```python
from build123d import *

# Parameters (mm, degrees)
SKETCH_1_R          = 2.5
EXTRUDE_1_DEPTH     = 3
SKETCH_2_R          = 2
EXTRUDE_2_DEPTH     = 3
SKETCH_3_R          = 0.25
CUT_EXTRUDE_1_DEPTH = 10


with BuildPart() as part:
    # Эскиз1 → Бобышка-Вытянуть1 (new body)
    with BuildSketch(Plane(origin=(0, 0, 0), x_dir=(1, 0, 0), z_dir=(0, 1, 0))):
        with Locations(Location((0, 0, 0), (0, 0, 270))):
            Circle(SKETCH_1_R)
    extrude(amount=EXTRUDE_1_DEPTH)

    # Эскиз2 → Бобышка-Вытянуть2 (add)
    with BuildSketch(Plane(origin=(0, 3, 0), x_dir=(1, 0, 0), z_dir=(0, 1, 0))):
        with Locations(Location((0, 0, 0), (0, 0, 270))):
            Circle(SKETCH_2_R)
    extrude(amount=EXTRUDE_2_DEPTH)

    # Эскиз3 → Вырез-Вытянуть1 (cut)
    with BuildSketch(Plane.XZ):
        with Locations(Location((0, -1.27, 0), (0, 0, 270))):
            Circle(SKETCH_3_R)
        with Locations(Location((1.27, 0, 0), (0, 0, 270))):
            Circle(SKETCH_3_R)
        with Locations(Location((-1.27, 0, 0), (0, 0, 270))):
            Circle(SKETCH_3_R)
    extrude(amount=-CUT_EXTRUDE_1_DEPTH, mode=Mode.SUBTRACT)


solid = part.part
```
Source: CAD feature listing. Evaluate the final solid. Frame: model axes, mm. A direction names the side the tool comes from. Give positions to 0.01 mm unless a question says otherwise; leave off trailing zeros. Order: outer loops, then holes, each group sorted by start corner. A loop starts at its lowest first (then second) coordinate and runs counter-clockwise, first axis right, second up.
(1) Section query C-C (y = 3.95). Return the cut outline in (x, z).
(2) Access query for faces 1 (the face through (-2, 4, 0)), 2 (the face through (0, 6, 0)). Directions: +Z, -Z, +X, -X, +Y, -Y. A direction counts if a zero-diameter tool reaches every point of the face in a straight line with its end or side. Return the directions, or none.
(3) Section query B-B (z = -1.27). Return the cut outline in (x, y), plus the area to 3 significant figures.
(4) Contact query for a flat-ended pin moving along its axis: P1, Ø1.5, axis at x = 1.5, z = 1.5, coming from the -Y side. Output: stop coordinate, or through.
(5) Material intervals for line 1 along X through (y, z) = (3.65, 0); line 2 along X through (y, z) = (2.3, -1.27); line 3 along Y through (x, z) = (2.1, -1.2), sorted ascending.
(6) Section query D-D (x = -1.65). Return the cut outline in (y, z), plus the area to 3 significant figures.
(7) Section query A-A (x = 0). Return the cut outline in (y, z).
Outcome:
1. outline: circle Ø4 at (0, 0); hole circle Ø0.5 at (-1.27, 0); hole circle Ø0.5 at (0, -1.27); hole circle Ø0.5 at (1.27, 0)
2. face 1: +Y
2. face 2: +Z, -Z, +X, -X, +Y
3. outline: (-2.15, 0) - (-0.25, 0) - (-0.25, 6) - (-1.55, 6) - (-1.55, 3) - (-2.15, 3) - close; (0.25, 0) - (2.15, 0) - (2.15, 3) - (1.55, 3) - (1.55, 6) - (0.25, 6) - close
3. area: 19.2 mm2
4. P1: stops at y = 0
5. line 1: x = -2 to -1.52, -1.02 to 1.02, 1.52 to 2
5. line 2: x = -2.15 to -0.25, 0.25 to 2.15
5. line 3: y = 0 to 3
6. outline: (0, -1.88) - (3, -1.88) - (3, -1.13) - (6, -1.13) - (6, 1.13) - (3, 1.13) - (3, 1.88) - (0, 1.88) - close
6. area: 18.1 mm2
7. outline: (0, -2.5) - (3, -2.5) - (3, -2) - (6, -2) - (6, -1.52) - (0, -1.52) - close; (0, -1.02) - (6, -1.02) - (6, 2) - (3, 2) - (3, 2.5) - (0, 2.5) - close
